The listing builds one solid part. Answer for the finished solid, in the listing's coordinates (mm). A direction names the side the tool comes from. Round coordinates to 2 decimals unless told otherwise and drop trailing zeros. Write each loop counter-clockwise with the first axis right and the second up, starting at its lowest first coordinate (ties: lowest second). Pieces come first, ordered by that corner, then holes. Notation, with made-up numbers: (0.5, 83.5) - (21.5, 83.5) arc R29 ccw to (21.5, 120.5) - close; hole circle Ø11 at (31.5, 12.5). An arc over 180 degrees is marked (long way). Answer in a Markdown table with one row per item.
from build123d import *

# Parameters (mm, degrees)
CUT_EXTRUDE1_START      = -1.8
CUT_EXTRUDE1_DEPTH      = 4.05
SKETCH6_R               = 1.5
CUT_EXTRUDE2_DEPTH      = 1
CUT_EXTRUDE2_DEPTH_BACK = 10


with BuildPart() as part:
    # Sketch4 → Revolve2 (revolve)
    with BuildSketch(Plane.XY):
        with BuildLine():
            Line((0, 13.692810861), (0, 0))
            Line((0, 0), (3.75, 0))
            Line((3.75, 0), (3.75, 13.692810861))
            ThreePointArc((3.75, 13.692810861), (4.557189139, 19.057189139), (0, 22))
            Line((0, 22), (0, 19.93))
            ThreePointArc((0, 19.93), (2.93, 17), (0, 14.07))
            Line((0, 14.07), (0, 13.692810861))
        make_face()
    revolve(axis=Axis((0, 26.788570074, 0), (0, -1, 0)))

    # Sketch5 → Cut-Extrude1 (cut)
    with BuildSketch(Plane(origin=(3.75, 0, 0), x_dir=(0, 0, -1), z_dir=(1, 0, 0)).offset(CUT_EXTRUDE1_START)):
        with BuildLine():
            Line((-3.75, 9.942810861), (3.75, 9.942810861))
            Line((3.75, 9.942810861), (3.75, 13.692810861))
            ThreePointArc((3.75, 13.692810861), (0, 22), (-3.75, 13.692810861))
            Line((-3.75, 13.692810861), (-3.75, 9.942810861))
        make_face()
    cut_extrude1 = extrude(amount=CUT_EXTRUDE1_DEPTH, mode=Mode.SUBTRACT)

    # Mirror2: Cut-Extrude1 across plane
    add(cut_extrude1.mirror(Plane(origin=(0, 0, 0), x_dir=(0, 0, 1), z_dir=(1, 0, 0))), mode=Mode.SUBTRACT)

    # Sketch6 → Cut-Extrude2 (cut, two sides)
    with BuildSketch(Plane.XZ) as cut_extrude2_sk:
        Circle(SKETCH6_R)
    extrude(amount=CUT_EXTRUDE2_DEPTH, mode=Mode.SUBTRACT)
    extrude(cut_extrude2_sk.sketch, amount=-CUT_EXTRUDE2_DEPTH_BACK, mode=Mode.SUBTRACT)


solid = part.part
(1) Find the intervals of material crossed by line 1 (Z direction, x = 0, y = 7.75); line 2 (X direction, y = 17.25, z = 3.25); line 3 (Y direction, x = 2.5, z = 2.25), in increasing order.
Checked values:
| item | result |
|---|---|
| line 1 | z = -3.75 to -1.5, 1.5 to 3.75 |
| line 2 | x = -1.95 to 1.95 |
| line 3 | y = 0 to 9.94 |
(2) Flat-ended cylindrical pins translate along their axes: pin 1 (2.5 mm diameter, centred on x = 0, z = 0, fed in from -Y); pin 2 (5 mm diameter, centred on y = 14.5, z = -1, fed in from +X); pin 3 (0.5 mm diameter, centred on x = -3, z = -0.5, fed in from +Y). Find the tip coordinate at first contact, or state that the pin passes through.
Checked values:
| item | result |
|---|---|
| pin 1 | stops at y = 10 |
| pin 2 | stops at x = 1.95 |
| pin 3 | stops at y = 9.94 |
(3) Section A-A (x = 0) is taken. Give the vertices of the cut face in (y, z).
Checked values:
| item | result |
|---|---|
| outline | (0, -3.75) - (13.69, -3.75) arc R5 ccw (long way) to (13.69, 3.75) - (0, 3.75) - (0, 1.5) - (10, 1.5) - (10, -1.5) - (0, -1.5) - close; hole circle Ø5.86 at (17, 0) |
(4) For faces 4 (the flat face through (0, 10, 0)), 5 (the flat face through (1.95, 14.6, 0.1)), 6 (the flat face through (-1.95, 14.6, 0.1)), determine the directions among +Z, -Z, +X, -X, +Y, -Y from which every point of the face is accessible in a straight line to the end or side of a thin tool.
Checked values:
| item | result |
|---|---|
| face 4 | -Y |
| face 5 | +Z, -Z, +X, +Y |
| face 6 | +Z, -Z, -X, +Y |
(5) Section B-B (z = 0) is taken. Give the vertices of the cut face in (x, y).
Checked values:
| item | result |
|---|---|
| outline | (-3.75, 0) - (-1.5, 0) - (-1.5, 10) - (1.5, 10) - (1.5, 0) - (3.75, 0) - (3.75, 9.94) - (1.95, 9.94) - (1.95, 14.81) arc R2.93 cw to (-1.95, 14.81) - (-1.95, 9.94) - (-3.75, 9.94) - close; (-1.95, 19.19) arc R2.93 cw to (1.95, 19.19) - (1.95, 21.6) arc R5 ccw to (-1.95, 21.6) - close |
(6) For a pull along Z with two mould halves and no side action, classify faces 1 (the cylindrical face through (-0.81, 5.42, -3.66)), 2 (the cylindrical face through (-1.5, 4.93, 0.07)), 3 (the flat face through (3, 9.943, 0)) as pulls with the +Z half, pulls with the -Z half, needs draft (parallel to the pull), parting line crosses it, or undercut.
Checked values:
| item | result |
|---|---|
| face 1 | parting line crosses it |
| face 2 | undercut |
| face 3 | needs draft |
(7) Section C-C (y = 17.25) is taken. Give the vertices of the cut face in (x, z), and give its area (3 significant figures).
Checked values:
| item | result |
|---|---|
| outline | (-1.95, -4.6) arc R4.99 ccw to (1.95, -4.6) - (1.95, -2.17) arc R2.92 cw to (-1.95, -2.17) - close; (-1.95, 2.17) arc R2.92 cw to (1.95, 2.17) - (1.95, 4.6) arc R4.99 ccw to (-1.95, 4.6) - close |
| area | 17.0 mm2 |
(8) Section D-D (y = 4.25) is taken. Give the vertices of the cut face in (x, z).
Checked values:
| item | result |
|---|---|
| outline | circle Ø7.5 at (0, 0); hole circle Ø3 at (0, 0) |
